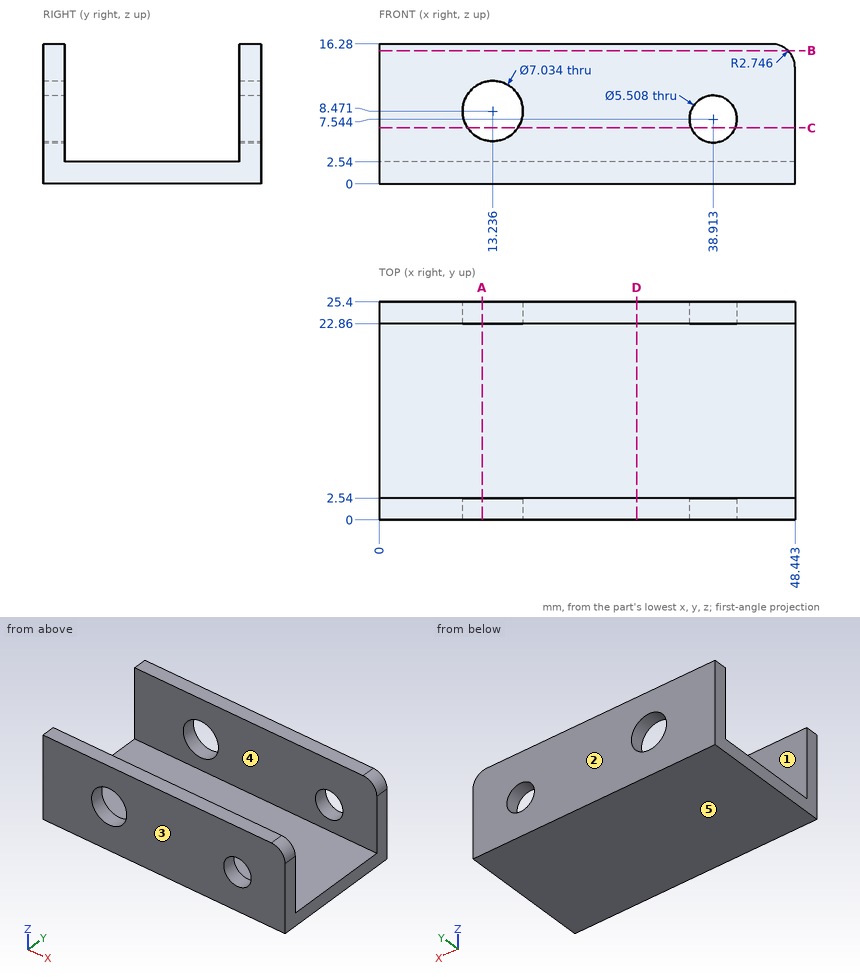
Design review of the part shown in the three views and the two pictorial views. Dimensions are in mm from the part's minimum x, y and z. A direction names the side the tool comes from. Give positions to 0.01 mm unless a question says otherwise; leave off trailing zeros. Loops run counter-clockwise (first coordinate to the right, second up) from the corner with the lowest first, then second, coordinate; pieces in that order, holes last. Notation, with made-up numbers: M -12,66.25 L 26,66.25 A23 cw 26,91.25 Z; hole C 82.25,80.5 d6. An arc over 180 degrees is marked long. Write item = value, one per line.
Q1. We need section C-C (z = 6.5). Give the boundary of the cut face in (x, y) (1 decimal).
Output values:
outline = M 0,0 L 10.3,0 L 10.3,2.5 L 0,2.5 Z; M 0,22.9 L 10.3,22.9 L 10.3,25.4 L 0,25.4 Z; M 16.1,0 L 36.4,0 L 36.4,2.5 L 16.1,2.5 Z; M 16.1,22.9 L 36.4,22.9 L 36.4,25.4 L 16.1,25.4 Z; M 41.5,0 L 48.4,0 L 48.4,2.5 L 41.5,2.5 Z; M 41.5,22.9 L 48.4,22.9 L 48.4,25.4 L 41.5,25.4 Z
Q2. We need section D-D (x = 30). Give the boundary of the cut face in (y, z).
Output values:
outline = M 0,0 L 25.4,0 L 25.4,16.28 L 22.86,16.28 L 22.86,2.54 L 2.54,2.54 L 2.54,16.28 L 0,16.28 Z
Q3. Draft analysis for pull direction Y (two halves, no side actions). For the marked faces 1, 2 and 3, state which applies: +Y half, -Y half, draft (parallel to the pull), parting line (faces both ways), or undercut.
Output values:
face_1 = undercut
face_2 = +Y half
face_3 = -Y half
Q4. For the marked faces 4 and 5, list the 3-axis set-ups (+Z, -Z, +X, -X, +Y, -Y) from which the entire face can be reached by the end or side of a thin tool; tool diameter is ignored.
Output values:
face_4 = +Z, +X, -X
face_5 = -Z, +X, -X, +Y, -Y
Q5. To check wall thickness, follow line 1 (Y direction, x = 21, z = 3.5); line 2 (Z direction, x = 23, y = 15). State the ranges of each line that lie inside material, in increasing order. Write a range as [from, to].
Output values:
line_1 = [0, 2.54], [22.86, 25.4]
line_2 = [0, 2.54]
Q6. We need section B-B (z = 15.5). Give the boundary of the cut face in (x, y).
Output values:
outline = M 0,0 L 47.61,0 L 47.61,2.54 L 0,2.54 Z; M 0,22.86 L 47.61,22.86 L 47.61,25.4 L 0,25.4 Z
Q7. Insertion check: pin 1 (5 mm diameter, centred on x = 31.5, y = 9.5, fed in from +Z). The pin has a flat end and moves straight along its axis. Give the tip position at first contact, or say it passes through.
Output values:
pin_1 = 2.54
Q8. We need section A-A (x = 12). Give the boundary of the cut face in (y, z).
Output values:
outline = M 0,0 L 25.4,0 L 25.4,5.18 L 22.86,5.18 L 22.86,2.54 L 2.54,2.54 L 2.54,5.18 L 0,5.18 Z; M 0,11.76 L 2.54,11.76 L 2.54,16.28 L 0,16.28 Z; M 22.86,11.76 L 25.4,11.76 L 25.4,16.28 L 22.86,16.28 Z
